```python
from build123d import *

# Parameters (mm, degrees)
PAD_DEPTH    = 6
SKETCH001_W  = 150
SKETCH001_H  = 73.5
POCKET_DEPTH = 3


with BuildPart() as part:
    # Sketch → Pad (new body)
    with BuildSketch(Plane.XZ):
        with BuildLine():
            Line((-52.75, 28.25), (52.75, 28.25))
            ThreePointArc((53.75, 27.25), (53.457107, 27.957107), (52.75, 28.25))
            Line((53.75, 27.25), (53.75, -27.25))
            ThreePointArc((52.75, -28.25), (53.457107, -27.957107), (53.75, -27.25))
            Line((52.75, -28.25), (-52.75, -28.25))
            ThreePointArc((-53.75, -27.25), (-53.457107, -27.957107), (-52.75, -28.25))
            Line((-53.75, -27.25), (-53.75, 27.25))
            ThreePointArc((-52.75, 28.25), (-53.457107, 27.957107), (-53.75, 27.25))
        make_face()
    extrude(amount=-PAD_DEPTH)

    # Sketch001 → Pocket (cut)
    with BuildSketch(Plane.XZ):
        Rectangle(SKETCH001_W, SKETCH001_H)
        with BuildLine():
            Line((-49, 24.5), (49, 24.5))
            ThreePointArc((50, 23.5), (49.707107, 24.207107), (49, 24.5))
            Line((50, 23.5), (50, -23.5))
            ThreePointArc((49, -24.5), (49.707107, -24.207107), (50, -23.5))
            Line((49, -24.5), (-49, -24.5))
            ThreePointArc((-50, -23.5), (-49.707107, -24.207107), (-49, -24.5))
            Line((-50, -23.5), (-50, 23.5))
            ThreePointArc((-49, 24.5), (-49.707107, 24.207107), (-50, 23.5))
        make_face(mode=Mode.SUBTRACT)
    extrude(amount=-POCKET_DEPTH, mode=Mode.SUBTRACT)


solid = part.part
```
The model under review builds one solid part; all positions refer to its coordinate system, in mm. A direction names the side the tool comes from. Give positions to 0.01 mm unless a question says otherwise; leave off trailing zeros. Write each loop counter-clockwise with the first axis right and the second up, starting at its lowest first coordinate (ties: lowest second). Pieces come first, ordered by that corner, then holes.
(1) Consider section B-B, the plane z = 21. Give the boundary of the cut face in (x, y).
(2) For P1, Ø1.5, axis at x = 8.5, y = 1, coming from the +Z side; P2, Ø3.5, axis at y = 1, z = -11, coming from the +X side; P3, Ø0.9, axis at x = -6, y = 1.5, coming from the -Z side, all flat-tipped, find the tip position at first contact; note any pin that passes through.
(3) Consider section A-A, the plane x = 33.5. Give the boundary of the cut face in (y, z).
(4) To check wall thickness, follow L1, parallel to Z at x = 27.5, y = 1.75; L2, parallel to X at y = 2.7, z = 6; L3, parallel to Y at x = -35, z = 26.5. State the ranges of each line that lie inside material, in increasing order.
(5) Tool access review of faces 1 (the flat face through (1, 1, -24.5)), 2 (the flat face through (-50, 1, 0)), 3 (the flat face through (50, 1, 0)), 4 (the flat face through (-4, 3, -25)), 5 (the flat face through (-1, 1, 24.5)): name each direction out of +Z, -Z, +X, -X, +Y, -Y from which nothing blocks a thin tool from reaching the whole face with its end or side.
Returned:
1. outline: (-53.75, 3) - (-50, 3) - (-50, 0) - (50, 0) - (50, 3) - (53.75, 3) - (53.75, 6) - (-53.75, 6) - close
2. P1: stops at z = 24.5
2. P2: stops at x = 50
2. P3: stops at z = -24.5
3. outline: (0, -24.5) - (3, -24.5) - (3, -28.25) - (6, -28.25) - (6, 28.25) - (3, 28.25) - (3, 24.5) - (0, 24.5) - close
4. L1: z = -24.5 to 24.5
4. L2: x = -50 to 50
4. L3: y = 3 to 6
5. face 1: -Z, +X, -X, -Y
5. face 2: +Z, -Z, -X, -Y
5. face 3: +Z, -Z, +X, -Y
5. face 4: -Y
5. face 5: +Z, +X, -X, -Y
